from build123d import *

# Parameters (mm, degrees)
ESQUISSE1_W        = 500
ESQUISSE1_H        = 500
BOSS_EXTRU_1_DEPTH = 250
COQUE1_T           = -10


with BuildPart() as part:
    # Esquisse1 → Boss.-Extru.1 (new body)
    with BuildSketch(Plane(origin=(0, 0, 0), x_dir=(1, 0, 0), z_dir=(0, 1, 0))):
        with Locations((104.080562725, 151.338562297)):
            Rectangle(ESQUISSE1_W, ESQUISSE1_H)
    extrude(amount=BOSS_EXTRU_1_DEPTH)

    # Coque1
    coque1_openings = [part.faces().sort_by_distance(p)[0] for p in [
        (104.080562725, 250, -151.338562297),
    ]]
    offset(amount=COQUE1_T, openings=coque1_openings, kind=Kind.INTERSECTION)


solid = part.part
Could you check a few things on this model? Use its own coordinates, in mm. A direction names the side the tool comes from. Round coordinates to 2 decimals unless told otherwise and drop trailing zeros. Order: outer loops, then holes, each group sorted by start corner. A loop starts at its lowest first (then second) coordinate and runs counter-clockwise, first axis right, second up.
Q1. Imagine slicing it at A-A, the plane y = 158.5. List the corners of the cut face in (x, z) for me, then the cut area to 3 significant figures.
Geometry says:
outline: (-145.92, -401.34) - (354.08, -401.34) - (354.08, 98.66) - (-145.92, 98.66) - close; hole (-135.92, -391.34) - (344.08, -391.34) - (344.08, 88.66) - (-135.92, 88.66) - close
area: 19,600 mm2
Q2. Imagine slicing it at C-C, the plane x = 151.5. List the corners of the cut face in (y, z) for me, then the cut area to 3 significant figures.
Geometry says:
outline: (0, -401.34) - (250, -401.34) - (250, -391.34) - (10, -391.34) - (10, 88.66) - (250, 88.66) - (250, 98.66) - (0, 98.66) - close
area: 9,800 mm2
Q3. I'm going to push a flat-ended pin straight in: P1, Ø4, axis at x = 111.5, z = 47, coming from the +Y side. Where does the tip first touch, or does it pass through?
Geometry says:
P1: stops at y = 10
Q4. Please list where these lines run through material, in increasing order: probe 1 along X at (y, z) = (32, -312.5); probe 2 along Z at (x, y) = (43.5, 67); probe 3 along Y at (x, z) = (-112, -235).
Geometry says:
probe 1: x = -145.92 to -135.92, 344.08 to 354.08
probe 2: z = -401.34 to -391.34, 88.66 to 98.66
probe 3: y = 0 to 10
Q5. Which directions (+Z, -Z, +X, -X, +Y, -Y) give clear straight access to the entire face, cutting with the end or side of a thin tool? Please do faces 4 (the face through (101, 128, 88.661)), 5 (the face through (-145.919, 123, -148)).
Geometry says:
face 4: +Y
face 5: +Z, -Z, -X, +Y, -Y
Q6. Thinking about a two-plate mould opening in X: for faces 1 (the face through (354.081, 123, -148)), 2 (the face through (101, 128, -391.339)), 3 (the face through (101, 0, -155)), which applies, released by +X, released by -X, zero draft, split by the parting line, or undercut?
Geometry says:
face 1: released by +X
face 2: undercut
face 3: zero draft
Q7. Imagine slicing it at B-B, the plane z = -355. List the corners of the cut face in (x, y) for me.
Geometry says:
outline: (-145.92, 0) - (354.08, 0) - (354.08, 250) - (344.08, 250) - (344.08, 10) - (-135.92, 10) - (-135.92, 250) - (-145.92, 250) - close
